Geometry check sheet. Reference: the model listing, model coordinates, mm. A direction names the side the tool comes from. Give positions to 0.01 mm unless a question says otherwise; leave off trailing zeros.
(1) Depth check by flat-ended pin: P1, Ø1.7, axis at y = 38.735, z = 1.27, coming from the -X side (3 decimals); P2, Ø1.4, axis at x = 1, y = 43, coming from the +Z side; P3, Ø4, axis at x = 5.5, z = -5, coming from the +Y side. Enter the tip coordinate at first touch or a pass-through.
(2) Tool access check on faces 1 (the flat face through (10.033, -49, -31)), 2 (the cylindrical face through (1, 38.37, 2.22)), 3 (the flat face through (-1.905, 23, 1)). Record the directions out of +Z, -Z, +X, -X, +Y, -Y that give a thin tool (end or side, any length) a straight path to the whole face; none if there is none.
(3) Thickness scan on line 1 along Z through (x, y) = (-8.2, 0); line 2 along X through (y, z) = (-15, 30.5) (3 decimals); line 3 along Y through (x, z) = (-5.25, 39). Record the ranges inside material, lowest first.
Autodesk Inventor part; units mm, degrees
ref_plane "YZ Plane" through (0, 0, 0) normal (1, 0, 0) x (0, 1, 0)
ref_plane "XZ Plane" through (0, 0, 0) normal (0, 1, 0) x (-1, 0, 0)
ref_plane "XY Plane" through (0, 0, 0) normal (0, 0, 1) x (1, 0, 0)
sketch "Sketch1" plane through (0, 0, 0) normal (0, 0, 1) x (1, 0, 0)
  line L0 (0, 0) -> (-10.033, 0)
  line L1 (-10.033, 0) -> (-10.033, -60.198)
  line L2 (-10.033, -60.198) -> (-4.953, -60.198)
  line L3 (-4.953, -60.198) -> (-4.953, -59.182)
  line L4 (-4.953, -59.182) -> (4.953, -59.182)
  line L5 (4.953, -59.182) -> (4.953, -60.198)
  line L6 (4.953, -60.198) -> (10.033, -60.198)
  line L7 (10.033, -60.198) -> (10.033, -57.658)
  line L8 (10.033, -57.658) -> (-10.033, -57.658)
  dimension "d0" = 10.033
  dimension "d1" = 60.198
  dimension "d2" = 5.08
  dimension "d3" = 1.016
  dimension "d4" = 9.906
  dimension "d5" = 1.016
  dimension "d6" = 5.08
  dimension "d7" = 2.54
revolve "Revolution1" add sketch "Sketch1" angle 360 about axis through (0, 0, 0) along (-1, 0, 0)
chamfer "Chamfer1" distance 1.016 angle 45 2 edges at (-4.953, 59.182, 0) (4.953, 59.182, 0)
sketch "Sketch2" plane through (0, 0, 0) normal (1, 0, 0) x (0, 1, 0)
  circle A0 centre (0, 0) radius 59.182
  circle A1 centre (0, 0) radius 19.05
  dimension "d12" = 118.364
  dimension "d13" = 38.1
extrude "Extrusion1" add sketch "Sketch2" along normal mid plane 3.81
chamfer "Chamfer2" distance 5.08 angle 45 2 edges at (1.905, 57.658, 0) (-1.905, 57.658, 0)
sketch "Sketch3" plane through (1.905, 0, 0) normal (1, 0, 0) x (0, 0, -1)
  line L0 (0, 0) -> (-29.3624, 0)
  dimension "d19" = 29.3624
hole "Hole1" at (1.905, 0, 29.3624) direction (-1, 0, 0) diameter 3.5052 end through all
pattern_circular "Circular Pattern1" count 3 over 360 about axis through (0, 0, 0) along (1, 0, 0) of "Hole1"
sketch "Sketch4" plane through (1.905, 0, 0) normal (1, 0, 0) x (0, 0, -1)
  circle A0 centre (0, 0) radius 32.385
  circle A1 centre (0, 0) radius 35.4838
  dimension "d30" = 64.77
  dimension "d31" = 70.9676
extrude "Extrusion2" cut sketch "Sketch4" against normal blind 1.8796
sketch "Sketch5" plane through (1.905, 0, 0) normal (1, 0, 0) x (0, 0, -1)
  line L0 (0, 0) -> (43.18, 0)
  line L1 (0, 0) -> (0, 25.4)
  line L2 (0, 0) -> (-43.18, 0)
  dimension "d34" = 43.18
  dimension "d35" = 25.4
hole "Hole2" at (1.905, 0, 43.18) at (1.905, 0, -43.18) direction (-1, 0, 0) diameter 4.064 end through all
sketch "Sketch6" plane through (1.905, 0, 0) normal (1, 0, 0) x (0, 0, -1)
  circle A0 centre (0, 0) radius 36.195
  line L0 (0, 36.195) -> (0, 37.465)
  line L1 (0, 37.465) -> (-3.175, 37.465)
  line L2 (-3.175, 37.465) -> (3.175, 37.465)
  line L3 (3.175, 37.465) -> (3.175, 50.165)
  line L4 (3.175, 50.165) -> (-3.175, 50.165)
  line L5 (-3.175, 50.165) -> (-3.175, 37.465)
  dimension "d43" = 72.39
  dimension "d44" = 1.27
  dimension "d45" = 3.175
  dimension "d46" = 6.35
  dimension "d47" = 12.7
extrude "Extrusion3" cut sketch "Sketch6" against normal blind 1.778 contours L1 L5 L4 L3 L2
sketch "Sketch7" plane through (0.127, 0, 0) normal (1, 0, 0) x (0, 0, -1)
  line L0 (3.175, 37.465) -> (-3.175, 37.465)
  line L1 (-3.175, 37.465) -> (-1.27, 37.465)
  line L2 (-1.27, 37.465) -> (-1.27, 38.735)
  line L3 (-1.27, 38.735) -> (-1.27, 41.275)
  line L4 (-1.27, 41.275) -> (-1.27, 43.815)
  line L5 (-1.27, 43.815) -> (-1.27, 46.355)
  line L6 (-1.27, 46.355) -> (-1.27, 48.895)
  line L7 (0, 37.465) -> (0, 50.165)
  line L8 (-3.175, 50.165) -> (3.175, 50.165)
  line L9 (1.27, 37.465) -> (1.27, 38.735)
  line L10 (1.27, 38.735) -> (1.27, 41.275)
  line L11 (1.27, 41.275) -> (1.27, 43.815)
  line L12 (1.27, 43.815) -> (1.27, 46.355)
  line L13 (1.27, 46.355) -> (1.27, 48.895)
  point P0 (0, 0)
  dimension "d50" = 1.905
  dimension "d51" = 1.27
  dimension "d52" = 2.54
  dimension "d53" = 2.54
  dimension "d54" = 2.54
  dimension "d55" = 2.54
  dimension "d56" = 12.7
hole "Hole3" at (0.127, 48.895, 1.27) at (0.127, 46.355, 1.27) at (0.127, 43.815, 1.27) at (0.127, 41.275, 1.27) at (0.127, 38.735, 1.27) at (0.127, 38.735, -1.27) at (0.127, 41.275, -1.27) at (0.127, 43.815, -1.27) at (0.127, 46.355, -1.27) at (0.127, 48.895, -1.27) direction (-1, 0, 0) diameter 1.27 end through all
fillet "Fillet1" radius 3.175 4 edges at (1.016, 37.465, -3.175) (1.016, 50.165, -3.175) (1.016, 50.165, 3.175) (1.016, 37.465, 3.175)
sketch "Sketch8" plane through (1.905, 0, 0) normal (1, 0, 0) x (0, 0, -1)
  circle A0 centre (0, -44.45) radius 6.1516
  point P0 (0, 0)
  dimension "d65" = 12.3031
  dimension "d66" = 44.45
extrude "Extrusion4" cut sketch "Sketch8" against normal blind 25.4
properties part number "Disc" material "Acetal Resin, Black"
Reply:
1. P1: stops at x = -1.905
1. P2: stops at z = 41.39
1. P3: stops at y = 60.12
2. face 1: +Z, -Z, +X, +Y, -Y
2. face 2: +X
2. face 3: -X
3. line 1: z = -60.2 to -57.66, 57.66 to 60.2
3. line 2: x = -1.905 to 0.025
3. line 3: y = -45.86 to -40.08, 40.08 to 45.86
